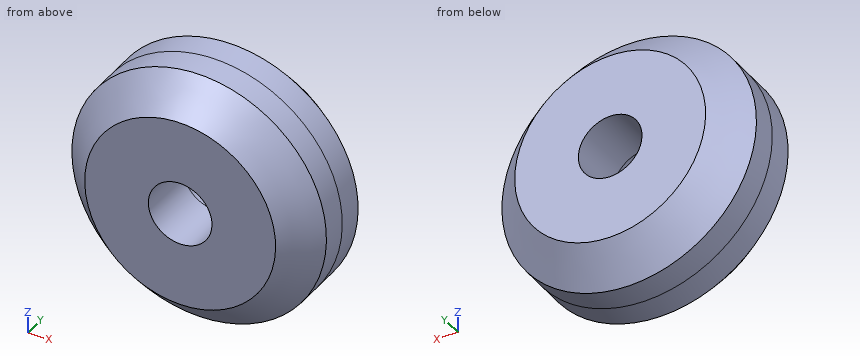
```python
from build123d import *


with BuildPart() as part:
    # Эскиз1 → Повернуть1 (revolve)
    with BuildSketch(Plane(origin=(0, 0, 0), x_dir=(0, 0, -1), z_dir=(1, 0, 0))):
        Polygon((3, 5.5), (9, 5.5), (12, 2.5), (12, 0), (3, 0), align=None)
    revolve_1 = revolve(axis=Axis((0, 0, 0), (0, 1, 0)))

    # Зеркальное отражение1: Повернуть1 across plane
    add(revolve_1.mirror(Plane.ZX))


solid = part.part
```
Model file for the job. Use its own axes, mm. Coordinates: 2 decimals unless noted, no trailing zeros. Order: outer loops, then holes, each group sorted by start corner. A loop starts at its lowest first (then second) coordinate and runs counter-clockwise, first axis right, second up. Notation, with made-up numbers: (74, 61) - (98, 61) arc R24 ccw to (98, 93) - close; hole circle Ø6 at (0, -38). An arc over 180 degrees is marked (long way). Return JSON: item names as keys, results as strings. Group by question number.
1) Probe line 1 (X direction, y = 2, z = 0); line 2 (Z direction, x = -1.75, y = 1); line 3 (Z direction, x = 2.25, y = -4.5). List the from-to ranges inside material, lowest first. Write a range as from..to.
2) Saw through at A-A, the plane z = 0. Write the cut outline in (x, y).
3) Saw through at B-B, the plane y = -3. Write the cut outline in (x, z), plus the area to 3 significant figures.
4) Saw through at C-C, the plane y = 1. Write the cut outline in (x, z), plus the area to 3 significant figures.
5) Flat gauge pins, fed straight in: P1, Ø4, axis at y = -2, z = -4.5, coming from the -X side; P2, Ø8, axis at x = 0, z = 0, coming from the -Y side; P3, Ø1.5, axis at x = 1, y = 0.5, coming from the -Z side; P4, Ø2, axis at y = -3, z = 1.5, coming from the -X side. Where does each tip first touch, or does it go through?
Values found:
{
 "1": {"line 1": "x = -12..-3, 3..12", "line 2": "z = -11.87..-2.44, 2.44..11.87", "line 3": "z = -9.74..-1.98, 1.98..9.74"},
 "2": {"outline": "(-12, -2.5) - (-9, -5.5) - (-3, -5.5) - (-3, 5.5) - (-9, 5.5) - (-12, 2.5) - close; (3, -5.5) - (9, -5.5) - (12, -2.5) - (12, 2.5) - (9, 5.5) - (3, 5.5) - close"},
 "3": {"outline": "circle Ø23 at (0, 0); hole circle Ø6 at (0, 0)", "area": "387 mm²"},
 "4": {"outline": "circle Ø24 at (0, 0); hole circle Ø6 at (0, 0)", "area": "424 mm²"},
 "5": {"P1": "stops at x = -11.74", "P2": "stops at y = -5.5", "P3": "stops at z = -12", "P4": "stops at x = -11.98"}
}
